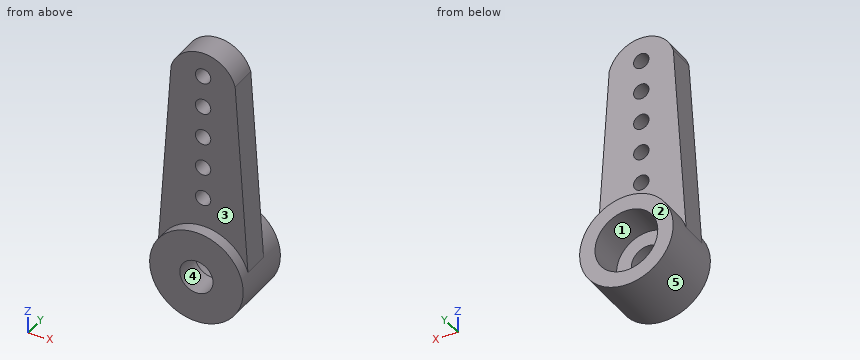
from build123d import *

# Parameters (mm, degrees)
SKETCH_3_R          = 3.65
EXTRUDE_1_DEPTH     = 2.5
SKETCH_4_R          = 2.45
CUT_EXTRUDE_1_DEPTH = 2.9
SKETCH_5_R          = 1.3
CUT_EXTRUDE_2_DEPTH = 6.920726307
EXTRUDE_2_DEPTH     = 2.1
SKETCH_7_R          = 0.6
CUT_EXTRUDE_3_DEPTH = 10


with BuildPart() as part:
    # 草图3 → 凸台-拉伸1 (new, symmetric)
    with BuildSketch(Plane(origin=(0, 0, 0), x_dir=(1, 0, 0), z_dir=(0, 1, 0))):
        with Locations(Location((0, 0, 0), (0, 0, 270))):
            Circle(SKETCH_3_R)
    extrude(amount=EXTRUDE_1_DEPTH, both=True)

    # 草图4 → 切除-拉伸1 (cut)
    with BuildSketch(Plane(origin=(0, 2.5, 0), x_dir=(1, 0, 0), z_dir=(0, 1, 0))):
        with Locations(Location((0, 0, 0), (0, 0, 270))):
            Circle(SKETCH_4_R)
    extrude(amount=-CUT_EXTRUDE_1_DEPTH, mode=Mode.SUBTRACT)

    # 草图5 → 切除-拉伸2 (cut, through all)
    with BuildSketch(Plane(origin=(0, -0.4, 0), x_dir=(1, 0, 0), z_dir=(0, 1, 0))):
        with Locations(Location((0, 0, 0), (0, 0, 270))):
            Circle(SKETCH_5_R)
    extrude(amount=-CUT_EXTRUDE_2_DEPTH, mode=Mode.SUBTRACT)

    # 草图6 → 凸台-拉伸2 (add)
    with BuildSketch(Plane(origin=(0, 0.5, 0), x_dir=(1, 0, 0), z_dir=(0, 1, 0))):
        with BuildLine():
            Line((3.5, -1.035615759), (2.5, -15.95))
            ThreePointArc((2.5, -15.95), (0, -17.85), (-2.5, -15.95))
            Line((-2.5, -15.95), (-3.5, -1.035615759))
            ThreePointArc((-3.5, -1.035615759), (0, -3.65), (3.5, -1.035615759))
        make_face()
    extrude(amount=-EXTRUDE_2_DEPTH)

    # 草图7 → 切除-拉伸3 (cut)
    with BuildSketch(Plane(origin=(0, 0.5, 0), x_dir=(1, 0, 0), z_dir=(0, 1, 0))):
        with Locations(Location((0, -15.95, 0), (0, 0, 270))):
            Circle(SKETCH_7_R)
        with Locations(Location((0, -13.45, 0), (0, 0, 270))):
            Circle(SKETCH_7_R)
        with Locations(Location((0, -10.95, 0), (0, 0, 270))):
            Circle(SKETCH_7_R)
        with Locations(Location((0, -8.45, 0), (0, 0, 270))):
            Circle(SKETCH_7_R)
        with Locations(Location((0, -5.95, 0), (0, 0, 270))):
            Circle(SKETCH_7_R)
    extrude(amount=-CUT_EXTRUDE_3_DEPTH, mode=Mode.SUBTRACT)


solid = part.part
Here's how the part is built. I have some questions about the finished solid (model axes, mm). Face numbers are marked on the shaded views. A direction names the side the tool comes from. Coordinates: 2 decimals unless noted, no trailing zeros. Write each loop counter-clockwise with the first axis right and the second up, starting at its lowest first coordinate (ties: lowest second). Pieces come first, ordered by that corner, then holes.
Item 1: I want a section at D-D on x = -3. Write out the boundary of the cut face in (y, z), and give its area (3 significant figures).
Item 2: I want a section at A-A on y = -1.35. Write out the boundary of the cut face in (x, z), and give its area (3 significant figures).
Item 3: Will these pins go through, and if not, where does the flat tip stop? pin 1 (3 mm diameter, centred on y = 1, z = 11, fed in from +X); pin 2 (3.5 mm diameter, centred on x = -0.5, z = 9, fed in from -Y); pin 3 (1.5 mm diameter, centred on x = -1, z = 0, fed in from +Y); pin 4 (1.6 mm diameter, centred on x = 0, z = 0, fed in from -Y).
Item 4: If we mould it in two halves opening along X, with no side actions, what happens to the marked faces 3, 4 and 5? For each: +X half, -X half, draft (parallel to the pull), parting line (faces both ways), or undercut.
Item 5: I want a section at B-B on z = 13.75. Write out the boundary of the cut face in (x, y), and give its area (3 significant figures).
Item 6: On a 3-axis mill with a long thin cutter (end or side, diameter ignored), from which of +Z, -Z, +X, -X, +Y, -Y can I reach the whole of each face in a straight line? I mean the marked faces 1 and 2. Say none if no direction works.
Item 7: If I drill on line 1 (X direction, y = -1.2, z = 8.45); line 2 (X direction, y = -0.3, z = 15.95); line 3 (Y direction, x = 1.5, z = 16), over which ranges is the centre line in solid material (lowest first)?
Item 8: I want a section at C-C on x = 1. Write out the boundary of the cut face in (y, z), and give its area (3 significant figures).
Findings below:
1. outline: (-2.5, -2.08) - (2.5, -2.08) - (2.5, 2.08) - (0.5, 2.08) - (0.5, 8.49) - (-1.6, 8.49) - (-1.6, 2.08) - (-2.5, 2.08) - close
1. area: 34.3 mm2
2. outline: (-3.5, 1.04) arc R3.65 ccw (long way) to (3.5, 1.04) - (2.5, 15.95) arc R2.59 ccw to (-2.5, 15.95) - close; hole circle Ø2.6 at (0, 0); hole circle Ø1.2 at (0, 5.95); hole circle Ø1.2 at (0, 8.45); hole circle Ø1.2 at (0, 10.95); hole circle Ø1.2 at (0, 13.45); hole circle Ø1.2 at (0, 15.95)
2. area: 114 mm2
3. pin 1: stops at x = 2.93
3. pin 2: stops at y = -1.6
3. pin 3: stops at y = -0.4
3. pin 4: passes through
4. face 3: draft
4. face 4: undercut
4. face 5: parting line
5. outline: (-2.65, -1.6) - (-0.52, -1.6) - (-0.52, 0.5) - (-2.65, 0.5) - close; (0.52, -1.6) - (2.65, -1.6) - (2.65, 0.5) - (0.52, 0.5) - close
5. area: 8.94 mm2
6. face 1: +Y
6. face 2: +Z, -Z, +X, -X, +Y
7. line 1: x = -3 to -0.6, 0.6 to 3
7. line 2: x = -2.5 to -0.6, 0.6 to 2.5
7. line 3: y = -1.6 to 0.5
8. outline: (-2.5, -3.51) - (2.5, -3.51) - (2.5, -2.24) - (-0.4, -2.24) - (-0.4, -0.83) - (-2.5, -0.83) - close; (-2.5, 0.83) - (-0.4, 0.83) - (-0.4, 2.24) - (2.5, 2.24) - (2.5, 3.51) - (0.5, 3.51) - (0.5, 17.65) - (-1.6, 17.65) - (-1.6, 3.51) - (-2.5, 3.51) - close
8. area: 48.3 mm2
